Autodesk Inventor part; units mm, degrees
ref_plane "YZ Plane" through (0, 0, 0) normal (1, 0, 0) x (0, 1, 0)
ref_plane "XZ Plane" through (0, 0, 0) normal (0, 1, 0) x (-1, 0, 0)
ref_plane "XY Plane" through (0, 0, 0) normal (0, 0, 1) x (1, 0, 0)
sketch "Sketch1" plane through (0, 0, 0) normal (0, 0, 1) x (1, 0, 0)
  line L0 (-50.8, -25.4) -> (50.8, -25.4)
  line L1 (50.8, -25.4) -> (50.8, 25.4)
  line L2 (50.8, 25.4) -> (-50.8, 25.4)
  line L3 (-50.8, 25.4) -> (-50.8, -25.4)
  line L4 (-50.8, -25.4) -> (50.8, 25.4) construction
  line L5 (50.8, -25.4) -> (-50.8, 25.4) construction
  point P0 (0, 0)
  dimension "d0" = 50.8
  dimension "d1" = 101.6
extrude "Extrusion1" add sketch "Sketch1" against normal blind 38.1
sketch "Sketch2" plane through (0, 0, 0) normal (0, 0, 1) x (1, 0, 0)
  line L0 (-50.8, 25.4) -> (50.8, 25.4)
  line L1 (50.8, -25.4) -> (-50.8, -25.4)
  line L2 (-25.4, 25.4) -> (0, 25.4)
  line L3 (0, 25.4) -> (0, -25.4)
  line L4 (0, -25.4) -> (-25.4, -25.4)
  line L5 (-25.4, -25.4) -> (-25.4, 25.4)
  line L6 (-50.8, 25.4) -> (-50.8, -25.4)
  point P0 (0, 0)
  dimension "d4" = 25.4
  dimension "d5" = 25.4
extrude "Extrusion2" cut sketch "Sketch2" against normal blind 25.4 contours L0 L3 L1 L5
sketch "Sketch3" plane through (0, 0, 0) normal (0, 0, 1) x (1, 0, 0)
  line L0 (0, 25.4) -> (0, -25.4)
  point P0 (0, 0)
  point P1 (31.75, 0)
  dimension "d8" = 31.75
hole "Hole1" at (31.75, 0, 0) direction (0, 0, -1) diameter 26.67 depth 31.75
sketch "Sketch4" plane through (31.75, 0, -31.75) normal (0, 0, 1) x (1, 0, 0)
  circle A0 centre (0, 0) radius 4.7625
  point P0 (-31.75, 0)
  dimension "d16" = 9.525
extrude "Extrusion3" cut sketch "Sketch4" against normal through all
sketch "Sketch5" plane through (-50.8, 25.4, -38.1) normal (0, 1, 0) x (1, 0, 0)
  line L0 (114.3, -38.1) -> (50.8, -38.1) construction
  line L1 (82.55, -38.1) -> (82.55, 0) construction
  line L2 (0, 0) -> (101.6, 0) construction
  line L3 (50.8, -12.7) -> (50.8, -38.1)
  line L4 (82.55, -9.2202) -> (82.55, -25.0952) construction
  line L5 (85.8266, -9.2202) -> (85.8266, -25.0952)
  line L6 (79.2734, -25.0952) -> (79.2734, -9.2202)
  arc A0 (85.8266, -9.2202) -> (79.2734, -9.2202) centre (82.55, -9.2202) ccw
  arc A1 (79.2734, -25.0952) -> (85.8266, -25.0952) centre (82.55, -25.0952) ccw
  point P0 (82.55, -15.5702)
  point P1 (82.55, -17.1577)
  dimension "d19" = 15.5702
  dimension "d44" = 31.75
  dimension "d64" = 6.35
  dimension "d65" = 6.5532
  dimension "d66" = 9.525
sketch "Sketch6" plane through (0, 0, -38.1) normal (0, 0, -1) x (-1, 0, 0)
  line L0 (25.4, 25.4) -> (0, 25.4) construction
  line L1 (12.7, 25.4) -> (12.7, -25.4) construction
  line L2 (-50.8, -25.4) -> (50.8, -25.4) construction
  point P0 (0, 0)
  point P1 (12.7, 12.7)
  point P2 (12.7, -12.7)
  dimension "d27" = 12.7
  dimension "d28" = 12.7
hole "Hole3" at (-12.7, 12.7, -38.1) at (-12.7, -12.7, -38.1) direction (0, 0, 1) diameter 5.1054 end through all
sketch "Sketch7" plane through (-50.8, -25.4, 0) normal (-1, 0, 0) x (0, 0, 1)
  line L0 (0, 50.8) -> (-38.1, 50.8) construction
  line L1 (-12.7, 50.8) -> (-12.7, 0) construction
  line L2 (0, 0) -> (-38.1, 0) construction
  point P0 (0, 25.4)
  point P1 (-25.4, 50.8)
  point P2 (-12.7, 25.4)
  dimension "d36" = 12.7
hole "Hole4" at (-50.8, 0, -12.7) direction (1, 0, 0) diameter 5.1054 end up to surface
sketch "Sketch8" plane through (0, 0, 0) normal (0, 0, 1) x (1, 0, 0)
  point P0 (0, 0)
sketch "Sketch9" plane through (0, 0, 0) normal (0, 0, 1) x (1, 0, 0)
  line L0 (-25.4, 25.4) -> (0, 25.4)
  line L1 (50.8, 25.4) -> (50.8, -25.4)
  line L2 (0, 25.4) -> (50.8, 25.4)
  line L3 (50.8, 25.4) -> (50.8, -25.4)
  line L4 (50.8, -25.4) -> (0, -25.4)
  line L5 (0, -25.4) -> (0, 25.4)
  circle A0 centre (31.75, 0) radius 13.335
  circle A1 centre (31.75, 0) radius 13.335
  point P0 (0, 0)
extrude "Extrusion4" add sketch "Sketch9" along normal blind 41.275
sketch "Sketch10" plane through (-50.8, 25.4, -38.1) normal (0, 1, 0) x (1, 0, 0)
  line L0 (77.7875, 0) -> (87.3125, 0) construction
  line L1 (82.55, 0) -> (82.55, -79.375) construction
  line L2 (50.8, -79.375) -> (101.6, -79.375) construction
  point P0 (50.8, -38.1)
  point P1 (82.55, -69.85)
  dimension "d47" = 9.525
hole "Hole5" at (31.75, 25.4, 31.75) direction (0, -1, 0) diameter 5.7912 end through all
sketch "Sketch11" plane through (0, 0, -38.1) normal (0, 0, -1) x (-1, 0, 0)
  circle A0 centre (-31.75, 0) radius 4.7625
  circle A1 centre (-31.75, 0) radius 6.35
  point P0 (0, 0)
  dimension "d55" = 12.7
extrude "Extrusion5" cut sketch "Sketch11" against normal blind 3.81
sketch "Sketch13" plane through (0, 0, 41.275) normal (0, 0, 1) x (1, 0, 0)
  line L0 (50.8, -25.4) -> (-50.8, -25.4)
  line L1 (0, 25.4) -> (0, -25.4)
  line L2 (50.8, -25.4) -> (0, -25.4)
  line L3 (0, -25.4) -> (0, 25.4)
  line L4 (0, 25.4) -> (50.8, 25.4)
  line L5 (50.8, 25.4) -> (50.8, -25.4)
  point P0 (0, 0)
extrude "Extrusion6" cut sketch "Sketch13" against normal blind 15.875
sketch "Sketch16" plane through (-50.8, 25.4, -38.1) normal (0, 1, 0) x (1, 0, 0)
  line L0 (25.4, -38.1) -> (0, -38.1)
  line L1 (25.4, -12.7) -> (20.32, -12.7)
  line L2 (20.32, -12.7) -> (20.32, -38.1)
  line L3 (20.32, -38.1) -> (25.4, -38.1)
  line L4 (25.4, -38.1) -> (25.4, -12.7)
  line L5 (50.8, -12.7) -> (50.8, -63.5)
  line L6 (101.6, -63.5) -> (50.8, -63.5)
  line L7 (50.8, -12.7) -> (55.88, -12.7)
  line L8 (55.88, -12.7) -> (55.88, -63.5)
  line L9 (55.88, -63.5) -> (50.8, -63.5)
  line L10 (50.8, -63.5) -> (50.8, -12.7)
  point P0 (50.8, -38.1)
  dimension "d60" = 5.08
  dimension "d61" = 5.08
extrude "Extrusion7" cut sketch "Sketch16" against normal through all
extrude "Extrusion8" cut sketch "Sketch5" against normal through all
equation "\"d0\" = height"
equation "\"d1\" = width"
equation "\"d2\" = depth"
equation "\"d6\" = slotFor1x1"
equation "\"d9\" = shaftDiameter + clearanceForRotation"
equation "\"d44\" = centerOfMotorShaft"
equation "\"width\" = 101.6"
equation "\"height\" = 50.8"
equation "\"depth\" = 38.1"
equation "\"shaftDiameter\" = 25.4"
equation "\"centerOfMotorShaft\" = 31.75"
equation "\"clearanceForRotation\" = 1.27"
equation "\"widthOfCChannel\" = 31.75"
properties part number "blockToSupportShaftAndPot" material "Aluminum 6061"
For this review, take the finished solid that the model builds, in its own axes (mm). A direction names the side the tool comes from. Give positions to 0.01 mm unless a question says otherwise; leave off trailing zeros. Order: outer loops, then holes, each group sorted by start corner. A loop starts at its lowest first (then second) coordinate and runs counter-clockwise, first axis right, second up. Notation, with made-up numbers: (-12.5, 38) -> (18.5, 38) arc R16 cw to (18.5, 57) -> close; hole circle Ø8 at (23, 62). An arc over 180 degrees is marked (long way). Write item = value, one per line.
1) We need section A-A, the plane y = 0. Count the separate pieces of the cut face and the enclosed holes in it, and give its area (3 significant figures).
Findings:
separate_pieces = 3
enclosed_holes = 0
area = 2,430 mm^2
2) Insertion check: pin 1 (8 mm diameter, centred on y = 0, z = -12.7, fed in from -X); pin 2 (10.5 mm diameter, centred on x = -14.5, y = -12.5, fed in from +Z); pin 3 (6 mm diameter, centred on x = -43.5, y = -10.5, fed in from +Z); pin 4 (13 mm diameter, centred on x = 36.5, y = 2, fed in from +Z). Each pin has a flat end and moves straight along its axis. Give the tip position at first contact, or say it passes through.
Findings:
pin_1 = -50.8
pin_2 = -25.4
pin_3 = 0
pin_4 = -31.75
3) We need section C-C, the plane x = -12.7. Give the boundary of the cut face in (y, z).
Findings:
outline = (-25.4, -38.1) -> (-15.25, -38.1) -> (-15.25, -25.4) -> (-25.4, -25.4) -> close; (-10.15, -38.1) -> (10.15, -38.1) -> (10.15, -25.4) -> (-10.15, -25.4) -> close; (15.25, -38.1) -> (25.4, -38.1) -> (25.4, -25.4) -> (15.25, -25.4) -> close
4) We need section D-D, the plane y = -18.5. Give the boundary of the cut face in (x, z), and give its area (3 significant figures).
Findings:
outline = (-50.8, -38.1) -> (50.8, -38.1) -> (50.8, 25.4) -> (5.08, 25.4) -> (5.08, -25.4) -> (-30.48, -25.4) -> (-30.48, 0) -> (-50.8, 0) -> close; hole (28.47, -28.88) arc R3.28 ccw to (35.03, -28.88) -> (35.03, -13) arc R3.28 ccw to (28.47, -13) -> close
area = 3,990 mm^2
5) We need section B-B, the plane z = -17. Give the boundary of the cut face in (x, y) (3 decimals), and give its area (3 significant figures).
Findings:
outline = (-50.8, -25.4) -> (-30.48, -25.4) -> (-30.48, 25.4) -> (-50.8, 25.4) -> close; (5.08, -25.4) -> (28.473, -25.4) -> (28.473, -12.926) arc R13.335 cw to (28.473, 12.926) -> (28.473, 25.4) -> (5.08, 25.4) -> close; (35.027, -25.4) -> (50.8, -25.4) -> (50.8, 25.4) -> (35.027, 25.4) -> (35.027, 12.926) arc R13.335 cw to (35.027, -12.926) -> close
area = 2,640 mm^2
6) Draft analysis for pull direction X (two halves, no side actions). For faces 4 (the face through (-50.8, 0, -19)), 5 (the face through (-1, 0, -38.1)), 6 (the face through (-13, 0, -25.4)), state which applies: pulls with the +X half, pulls with the -X half, needs draft (parallel to the pull), parting line crosses it, or undercut.
Findings:
face_4 = pulls with the -X half
face_5 = needs draft
face_6 = undercut
7) To check wall thickness, follow L1, parallel to Y at x = -12.7, z = -34.5; L2, parallel to X at y = 13, z = -15.5; L3, parallel to X at y = 0, z = -13.5 (3 decimals). State the ranges of each line that lie inside material, in increasing order. Write a range as from..to.
Findings:
L1 = -25.4..-15.25, -10.15..10.15, 15.25..25.4
L2 = -50.8..-30.48, 5.08..28.47, 35.03..50.8
L3 = 5.08..18.415, 45.085..50.8
8) For faces 1 (the face through (24, 0, -31.75)), 2 (the face through (25.693, 1.907, -36.222)), 3 (the face through (-30.48, 0, -16)), list the 3-axis set-ups (+Z, -Z, +X, -X, +Y, -Y) from which the entire face can be reached by the end or side of a thin tool; tool diameter is ignored.
Findings:
face_1 = +Z
face_2 = -Z
face_3 = +Z, +Y, -Y
